```python
from build123d import *

# Parameters (mm, degrees)
CUT_EXTRUDE1_REACH       = 154.4
CUT_EXTRUDE1_END_RADIUS  = 152.4
SKETCH2_R                = 25.4
BOSS_EXTRUDE3_REACH      = 611.6
BOSS_EXTRUDE3_END_RADIUS = 152.4
SKETCH4_R                = 31.75
SKETCH4_R_2              = 25.4
CUT_EXTRUDE2_REACH       = 713.2
CUT_EXTRUDE2_END_RADIUS  = 146.05
SKETCH5_R                = 15.875
BOSS_EXTRUDE4_REACH      = 713.2
BOSS_EXTRUDE4_END_RADIUS = 152.4
SKETCH6_R                = 22.225
SKETCH6_R_2              = 15.875


with BuildPart() as part:
    # Sketch1 → Revolve1 (revolve)
    with BuildSketch(Plane.XY, mode=Mode.PRIVATE) as revolve1_sk:
        with BuildLine():
            Line((-152.4, 101.6), (-152.4, -101.6))
            ThreePointArc((-152.4, -101.6), (-107.763073453, -209.363073453), (0, -254))
            Line((0, -254), (0, -247.65))
            ThreePointArc((0, -247.65), (-103.272945392, -204.872945392), (-146.05, -101.6))
            Line((-146.05, -101.6), (-146.05, 101.6))
            ThreePointArc((-146.05, 101.6), (-103.272945392, 204.872945392), (0, 247.65))
            Line((0, 247.65), (0, 254))
            ThreePointArc((0, 254), (-107.763073453, 209.363073453), (-152.4, 101.6))
        make_face()
    revolve(revolve1_sk.sketch.rotate(Axis((0, -254, 0), (0, 1, 0)), 180), axis=Axis((0, -254, 0), (0, 1, 0)))  # turned: the seam where the file's is

    # Cut-Extrude1: up to this cylinder (the profile starts inside it)
    cut_extrude1_end = Plane(origin=(0, 0, 0), z_dir=(0, -1, 0)) * Cylinder(CUT_EXTRUDE1_END_RADIUS, 614.6, mode=Mode.PRIVATE)
    # Sketch2 → Cut-Extrude1 (cut, up to the surface)
    with BuildSketch(Plane(origin=(0, 0, 0), x_dir=(0, 0, -1), z_dir=(1, 0, 0)), mode=Mode.PRIVATE) as cut_extrude1_sk1:
        Circle(SKETCH2_R)
    cut_extrude1_tool1 = extrude(cut_extrude1_sk1.sketch, amount=-CUT_EXTRUDE1_REACH, mode=Mode.PRIVATE) & cut_extrude1_end
    add(cut_extrude1_tool1.solids().sort_by_distance((0, 0, 0))[0], mode=Mode.SUBTRACT)

    # Boss-Extrude3: up to this cylinder (the profile starts outside it)
    boss_extrude3_end = Plane(origin=(0, 0, 0), z_dir=(0, -1, 0)) * Cylinder(BOSS_EXTRUDE3_END_RADIUS, 1529, mode=Mode.PRIVATE)
    # Sketch4 → Boss-Extrude3 (add, up to the surface)
    with BuildSketch(Plane(origin=(-457.2, 0, 0), x_dir=(0, 0, -1), z_dir=(1, 0, 0)), mode=Mode.PRIVATE) as boss_extrude3_sk1:
        with Locations(Location((0, 0, 0), (0, 0, 180))):  # turned: the seam where the file's is
            Circle(SKETCH4_R)
        Circle(SKETCH4_R_2, mode=Mode.SUBTRACT)
    boss_extrude3_tool1 = extrude(boss_extrude3_sk1.sketch, amount=BOSS_EXTRUDE3_REACH, mode=Mode.PRIVATE) - boss_extrude3_end
    add(boss_extrude3_tool1.solids().sort_by_distance((-457.2, 0, -30.851974))[0])

    # Cut-Extrude2: up to this sphere (the profile starts outside it)
    cut_extrude2_end = Location((0, -101.6, 0)) * Sphere(CUT_EXTRUDE2_END_RADIUS, mode=Mode.PRIVATE)
    # Sketch5 → Cut-Extrude2 (cut, up to the surface)
    with BuildSketch(Plane(origin=(0, -457.2, 0), x_dir=(1, 0, 0), z_dir=(0, 1, 0)), mode=Mode.PRIVATE) as cut_extrude2_sk1:
        with Locations(Location((0, 0, 0), (0, 0, 270))):  # turned: the seam where the file's is
            Circle(SKETCH5_R)
    cut_extrude2_tool1 = extrude(cut_extrude2_sk1.sketch, amount=CUT_EXTRUDE2_REACH, mode=Mode.PRIVATE) - cut_extrude2_end
    add(cut_extrude2_tool1.solids().sort_by_distance((0, -457.2, 0))[0], mode=Mode.SUBTRACT)

    # Boss-Extrude4: up to this sphere (the profile starts outside it)
    boss_extrude4_end = Location((0, -101.6, 0)) * Sphere(BOSS_EXTRUDE4_END_RADIUS, mode=Mode.PRIVATE)
    # Sketch6 → Boss-Extrude4 (add, up to the surface)
    with BuildSketch(Plane(origin=(0, -457.2, 0), x_dir=(1, 0, 0), z_dir=(0, 1, 0)), mode=Mode.PRIVATE) as boss_extrude4_sk1:
        with Locations(Location((0, 0, 0), (0, 0, 270))):  # turned: the seam where the file's is
            Circle(SKETCH6_R)
        with Locations(Location((0, 0, 0), (0, 0, 270))):  # turned: the seam where the file's is
            Circle(SKETCH6_R_2, mode=Mode.SUBTRACT)
    boss_extrude4_tool1 = extrude(boss_extrude4_sk1.sketch, amount=BOSS_EXTRUDE4_REACH, mode=Mode.PRIVATE) - boss_extrude4_end
    add(boss_extrude4_tool1.solids().sort_by_distance((0, -457.2, -21.596382))[0])


solid = part.part
```
The listing builds one solid part. Answer for the finished solid, in the listing's coordinates (mm). A direction names the side the tool comes from. Coordinates: 2 decimals unless noted, no trailing zeros. Loops run counter-clockwise (first coordinate to the right, second up) from the corner with the lowest first, then second, coordinate; pieces in that order, holes last. Notation, with made-up numbers: (77.5, -26) -> (109.5, -26) arc R11 cw to (109.5, -16) -> close; hole circle Ø10 at (18, 62.25). An arc over 180 degrees is marked (long way). Use one line per item in the form item = value. Start each with the question number.
Item 1: The part is cut by section C-C on y = 0. Determine the outline of the cut face in (x, z), then the cut area to 3 significant figures.
Item 2: A tool of negligible diameter and unlimited length cuts with its end or side. For faces 4 (the face through (-457.2, -21.3, -14.3)), 5 (the face through (-15.497, -353.465, -3.441)), 6 (the face through (-305.285, 30.995, -6.883)), from which of +Z, -Z, +X, -X, +Y, -Y can it reach the whole face along a straight path? Write none if from no direction.
Item 3: The part is cut by section D-D on x = -81. Determine the outline of the cut face in (y, z).
Item 4: The mould has two halves that part along Y. Classify faces 1 (the face through (18.74, -356.22, 11.95)), 2 (the face through (-15, -457.2, 10)), 3 (the face through (139.306, 1.422, -43.869)): released by +Y, released by -Y, zero draft, split by the parting line, or undercut.
Item 5: Flat-ended cylindrical pins translate along their axes: pin 1 Ø12 at (y, z) = (70.5, 53.5) entering from +X; pin 2 Ø1.5 at (y, z) = (-325, 13.5) entering from +X; pin 3 Ø6 at (x, y) = (49.5, -232.5) entering from +Z. Find the tip coordinate at first contact, or state that the pin passes through.
Item 6: Consider L1, parallel to Y at x = -258, z = 0; L2, parallel to X at y = -327, z = 0 (3 decimals). Determine where each line is inside the solid, lowest interval first. Write a range as [from, to].
Item 7: The part is cut by section A-A on x = 0. Determine the outline of the cut face in (y, z) (3 decimals).
Item 8: The part is cut by section B-B on z = 0. Determine the outline of the cut face in (x, y) (3 decimals).
Answer key:
q1.outline = (-457.2, -31.75) -> (-149.06, -31.75) arc R152.4 ccw (long way) to (-149.06, 31.75) -> (-457.2, 31.75) -> (-457.2, 25.4) -> (-143.82, 25.4) arc R146.05 cw (long way) to (-143.82, -25.4) -> (-457.2, -25.4) -> close
q1.area = 9,540 mm2
q2.face_4 = +Z, -Z, -X, +Y, -Y
q2.face_5 = -Y
q2.face_6 = -X
q3.outline = (-101.6, -129.09) -> (101.6, -129.09) arc R129.09 ccw to (101.6, 129.09) -> (-101.6, 129.09) arc R129.09 ccw to start; hole (-101.6, -121.53) -> (101.6, -121.53) arc R121.53 ccw to (101.6, 121.53) -> (-101.6, 121.53) arc R121.53 ccw to start
q4.face_1 = zero draft
q4.face_2 = released by -Y
q4.face_3 = undercut
q5.pin_1 = 144.81
q5.pin_2 = 18.2
q5.pin_3 = 66.87
q6.L1 = [-31.75, -25.4], [25.4, 31.75]
q6.L2 = [-22.225, -15.875], [15.875, 22.225]
q7.outline = (-457.2, -22.225) -> (-252.371, -22.225) arc R152.4 ccw to (-101.6, -152.4) -> (101.6, -152.4) arc R152.4 ccw to (101.6, 152.4) -> (-101.6, 152.4) arc R152.4 ccw to (-252.371, 22.225) -> (-457.2, 22.225) -> (-457.2, 15.875) -> (-246.785, 15.875) arc R146.05 cw to (-101.6, 146.05) -> (101.6, 146.05) arc R146.05 cw to (101.6, -146.05) -> (-101.6, -146.05) arc R146.05 cw to (-246.785, -15.875) -> (-457.2, -15.875) -> close
q8.outline = (-457.2, -31.75) -> (-152.4, -31.75) -> (-152.4, -101.6) arc R152.4 ccw to (-22.225, -252.371) -> (-22.225, -457.2) -> (-15.875, -457.2) -> (-15.875, -246.785) arc R146.05 cw to (-146.05, -101.6) -> (-146.05, -25.4) -> (-457.2, -25.4) -> close; (-457.2, 25.4) -> (-146.05, 25.4) -> (-146.05, 101.6) arc R146.05 cw to (146.05, 101.6) -> (146.05, -101.6) arc R146.05 cw to (15.875, -246.785) -> (15.875, -457.2) -> (22.225, -457.2) -> (22.225, -252.371) arc R152.4 ccw to (152.4, -101.6) -> (152.4, 101.6) arc R152.4 ccw to (-152.4, 101.6) -> (-152.4, 31.75) -> (-457.2, 31.75) -> close
